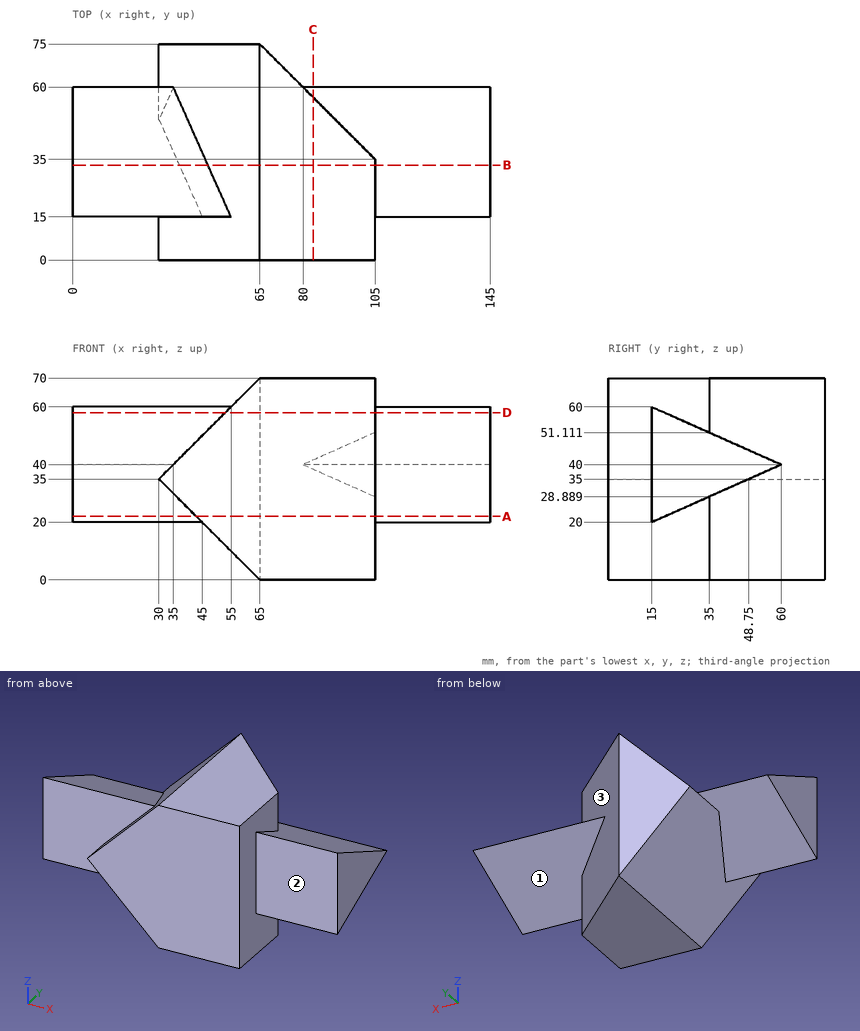
Geometry check sheet. Reference: drawing and pictorial views, mm from the part's lowest x, y, z. A direction names the side the tool comes from. Round coordinates to 2 decimals unless told otherwise and drop trailing zeros. Loops run counter-clockwise (first coordinate to the right, second up) from the corner with the lowest first, then second, coordinate; pieces in that order, holes last. Notation, with made-up numbers: (60.25, -28) - (114.25, -28) arc R24 ccw to (114.25, -1) - close; hole circle Ø9 at (17.25, 81.5). An arc over 180 degrees is marked (long way). Use a Markdown table: item, result.
Q1. Cross-section at C-C on x = 83.5. Record the cut outline in (y, z), plus the area to 3 significant figures.
Solutions:
| item | result |
|---|---|
| outline | (0, 0) - (56.5, 0) - (56.5, 38.44) - (60, 40) - (56.5, 41.56) - (56.5, 70) - (0, 70) - close |
| area | 3,960 mm2 |
Q2. Cross-section at B-B on y = 33. Record the cut outline in (x, z), plus the area to 3 significant figures.
Solutions:
| item | result |
|---|---|
| outline | (0, 28) - (37, 28) - (65, 0) - (105, 0) - (105, 28) - (145, 28) - (145, 52) - (105, 52) - (105, 70) - (65, 70) - (47, 52) - (0, 52) - close |
| area | 5,870 mm2 |
Q3. Go/stop test with flat-tipped pins: P1, Ø4, axis at x = 57.5, y = 54.5, coming from the -Z side; P2, Ø2, axis at x = 88, z = 35, coming from the +Y side; P3, Ø8, axis at x = 40, y = 24, coming from the +Z side. Record where each tip stops, or that it passes through.
Solutions:
| item | result |
|---|---|
| P1 | stops at z = 5.5 |
| P2 | stops at y = 53 |
| P3 | stops at z = 57.78 |
Q4. Cross-section at A-A on z = 22. Record the cut outline in (x, y).
Solutions:
| item | result |
|---|---|
| outline | (0, 15) - (43, 15) - (43, 0) - (105, 0) - (105, 15) - (145, 15) - (145, 19.5) - (105, 19.5) - (105, 35) - (65, 75) - (43, 75) - (43, 19.5) - (0, 19.5) - close |
Q5. Material ranges on line 1 (Z direction, x = 54.5, y = 58); line 2 (Y direction, x = 123.5, z = 31.5) (1 decimal); line 3 (Y direction, x = 89, z = 47), recorded low to high.
Solutions:
| item | result |
|---|---|
| line 1 | z = 10.5 to 59.5 |
| line 2 | y = 15 to 40.9 |
| line 3 | y = 0 to 51 |
Q6. Cross-section at D-D on z = 58. Record the cut outline in (x, y), plus the area to 3 significant figures.
Solutions:
| item | result |
|---|---|
| outline | (0, 15) - (53, 15) - (53, 0) - (105, 0) - (105, 15) - (145, 15) - (145, 19.5) - (105, 19.5) - (105, 35) - (65, 75) - (53, 75) - (53, 19.5) - (0, 19.5) - close |
| area | 3,520 mm2 |
Q7. Access from +Z, -Z, +X, -X, +Y, -Y to the whole of each face (thin tool, end or side, straight path). Record for the marked faces 1, 2 and 3.
Solutions:
| item | result |
|---|---|
| face 1 | -Z, +X, +Y |
| face 2 | +Z, -Z, +X, -Y |
| face 3 | +X, +Y |
